Work out the finished part from the listing and answer in its coordinate system (mm). A direction names the side the tool comes from. Round coordinates to 2 decimals unless told otherwise and drop trailing zeros. Loops run counter-clockwise (first coordinate to the right, second up) from the corner with the lowest first, then second, coordinate; pieces in that order, holes last.
```python
from build123d import *

# Parameters (mm, degrees)
F1_DEPTH = 63.5
F2_DEPTH = 7.9375
F0_W     = 25.4
F0_H     = 19.05
F3_DEPTH = 38.1


with BuildPart() as f1:
    # F0 (on Front) → F1 (new body, symmetric)
    with BuildSketch(Plane.XZ):
        Polygon((-41.275, 9.525), (-41.275, -9.525), (41.275, -9.525), (41.275, 9.525), (22.225, 9.525), align=None)
    extrude(amount=F1_DEPTH, both=True)

    # F0 (on Front) → F2 (join, symmetric)
    with BuildSketch(Plane.XZ):
        with BuildLine():
            add(Edge.make_bspline(
                [(-41.275, 9.525), (-19.269418, 48.490915), (8.980925, 77.770598), (57.15, 61.9252)],
                knots=[0, 0, 0, 0, 111.504536, 111.504536, 111.504536, 111.504536], degree=3))
            Line((-41.275, 9.525), (22.225, 9.525))
            Line((22.225, 9.525), (22.225, 27.0002))
            ThreePointArc((22.225, 27.0002), (32.454296, 51.695904), (57.15, 61.9252))
        make_face()
    extrude(amount=F2_DEPTH, both=True)

    # F0 (on Front) → F3 (join, symmetric)
    with BuildSketch(Plane.XZ):
        with BuildLine():
            Line((22.225, 9.525), (41.275, 9.525))
            Line((41.275, 9.525), (41.275, 27.0002))
            ThreePointArc((41.275, 27.0002), (45.92468, 38.22552), (57.15, 42.8752))
            Line((57.15, 42.8752), (60.325, 42.8752))
            Line((60.325, 42.8752), (60.325, 61.9252))
            Line((60.325, 61.9252), (57.15, 61.9252))
            ThreePointArc((57.15, 61.9252), (32.454296, 51.695904), (22.225, 27.0002))
            Line((22.225, 27.0002), (22.225, 9.525))
        make_face()
        with Locations((73.025, 52.4002)):
            Rectangle(F0_W, F0_H)
    extrude(amount=F3_DEPTH, both=True)

    # F0 (on Front) → F4 (revolve)
    with BuildSketch(Plane.XZ):
        Polygon((85.725, 66.675), (85.725, 61.9252), (85.725, 42.8752), (85.725, 38.1), (111.125, 38.1), (111.125, 66.675), align=None)
    revolve(axis=Axis((85.725, 0, 52.4002), (0, 0, -1)))


solid = f1.part
```
1. Given pin 1 (2 mm diameter, centred on y = -33.5, z = 49.5, fed in from +X) (3 decimals); pin 2 (2 mm diameter, centred on x = 21.5, z = 27, fed in from -Y); pin 3 (2 mm diameter, centred on y = 0, z = 36.5, fed in from -X); pin 4 (19 mm diameter, centred on y = 22, z = 15, fed in from -X) (3 decimals), each flat-ended and moving along its own axis, determine where each tip first touches the part or whether it passes through.
Answer key:
pin 1: stops at x = 85.725
pin 2: stops at y = -38.1
pin 3: stops at x = -24.1
pin 4: stops at x = -41.275
2. Determine the mould class of faces 4 (the face through (1, 35, 9.525)), 5 (the face through (32.73, 22.81, 51.97)), 6 (the face through (61.7, -9, 42.875)), 7 (the face through (85.725, -32, 52)) for opening direction X: +X half, -X half, draft (parallel to the pull), parting line (faces both ways), or undercut.
Answer key:
face 4: draft
face 5: -X half
face 6: undercut
face 7: +X half
3. Consider probe 1 along Y at (x, z) = (28, 60.5); probe 2 along Z at (x, y) = (11.5, 15.5) (3 decimals); probe 3 along X at (y, z) = (-1.5, 38.5). Determine where each line is inside the solid, lowest interval first.
Answer key:
probe 1: y = -7.94 to 7.94
probe 2: z = -9.525 to 9.525
probe 3: x = -21.62 to 46.21, 60.37 to 111.08
4. Find section B-B (x = 73). Write down the section's boundary in (y, z) (3 decimals), then the cut area to 3 significant figures.
Answer key:
outline: (-38.1, 42.875) - (-21.983, 42.875) - (-21.983, 38.1) - (21.983, 38.1) - (21.983, 42.875) - (38.1, 42.875) - (38.1, 61.925) - (21.983, 61.925) - (21.983, 66.675) - (-21.983, 66.675) - (-21.983, 61.925) - (-38.1, 61.925) - close
area: 1,870 mm2
5. Which of the six approach directions +Z, -Z, +X, -X, +Y, -Y give full straight-line access (tool end or side, diameter ignored) to faces 1 (the face through (22.225, 23, 18)), 2 (the face through (86, 0, 38.1)), 3 (the face through (46, -38.1, 42))?
Answer key:
face 1: +Z, -X, +Y
face 2: -Z, +X, +Y, -Y
face 3: +Z, +X, -X, -Y
6. Find section C-C (y = -48.5). Write down the section's boundary in (x, z) (3 decimals), then the cut area to 3 significant figures.
Answer key:
outline: (-41.275, -9.525) - (41.275, -9.525) - (41.275, 9.525) - (-41.275, 9.525) - close
area: 1,570 mm2
7. Find section A-A (y = -30). Write down the section's boundary in (x, z) (3 decimals).
Answer key:
outline: (-41.275, -9.525) - (41.275, -9.525) - (41.275, 27) arc R15.875 cw to (57.15, 42.875) - (85.725, 42.875) - (85.725, 61.925) - (57.15, 61.925) arc R34.925 ccw to (22.225, 27) - (22.225, 9.525) - (-41.275, 9.525) - close
